```python
from build123d import *

# Parameters (mm, degrees)
SKETCH1_R                = 12.75
BOSS_EXTRUDE1_DEPTH      = 13
SKETCH2_R                = 3.3
BOSS_EXTRUDE2_DEPTH      = 1
SKETCH3_R                = 2.5
BOSS_EXTRUDE3_DEPTH      = 10.5
SKETCH4_R                = 5
BOSS_EXTRUDE4_DEPTH      = 2
BOSS_EXTRUDE5_START      = 10.5
SKETCH5_R                = 2.5
BOSS_EXTRUDE5_DEPTH      = 10.5
CHAMFER1_SIZE            = 1
BOSS_EXTRUDE6_REACH      = 32.42
BOSS_EXTRUDE6_END_RADIUS = 22.75
SKETCH6_R                = 2.2


with BuildPart() as part:
    # Sketch1 → Boss-Extrude1 (new body)
    with BuildSketch(Plane(origin=(0, 0, 0), x_dir=(1, 0, 0), z_dir=(0, 1, 0))):
        with Locations(Location((0, 0, 0), (0, 0, 90))):
            Circle(SKETCH1_R)
    extrude(amount=BOSS_EXTRUDE1_DEPTH)

    # Sketch2 → Boss-Extrude2 (add)
    with BuildSketch(Plane(origin=(0, 13, 0), x_dir=(1, 0, 0), z_dir=(0, 1, 0))):
        with Locations(Location((0, 0, 0), (0, 0, 270))):
            Circle(SKETCH2_R)
    extrude(amount=BOSS_EXTRUDE2_DEPTH)

    # Sketch3 → Boss-Extrude3 (add)
    with BuildSketch(Plane(origin=(0, 14, 0), x_dir=(1, 0, 0), z_dir=(0, 1, 0))):
        with Locations(Location((0, 0, 0), (0, 0, 90))):
            Circle(SKETCH3_R)
    extrude(amount=BOSS_EXTRUDE3_DEPTH)

    # Sketch4 → Boss-Extrude4 (add)
    with BuildSketch(Plane.XZ):
        with Locations(Location((0, 0, 0), (0, 0, 270))):
            Circle(SKETCH4_R)
    extrude(amount=BOSS_EXTRUDE4_DEPTH)

    # Sketch5 → Boss-Extrude5 (add)
    with BuildSketch(Plane.XZ.offset(2).offset(BOSS_EXTRUDE5_START)):
        with Locations(Location((0, 0, 0), (0, 0, 270))):
            Circle(SKETCH5_R)
    extrude(amount=-BOSS_EXTRUDE5_DEPTH)

    # Chamfer1
    chamfer1_edges = [part.edges().sort_by_distance(p)[0] for p in [
        (0, 24.5, 2.5),
        (0, -12.5, 2.5),
    ]]
    chamfer(chamfer1_edges, length=CHAMFER1_SIZE)

    # Boss-Extrude6: up to this cylinder (the profile starts inside it)
    boss_extrude6_end = Plane(origin=(0, 3.7, 0), z_dir=(0, -1, 0)) * Cylinder(BOSS_EXTRUDE6_END_RADIUS, 111.34, mode=Mode.PRIVATE)
    # Sketch6 → Boss-Extrude6 (add, up to the surface)
    with BuildSketch(Plane(origin=(0, 0, 0), x_dir=(0, 0, -1), z_dir=(1, 0, 0)), mode=Mode.PRIVATE) as boss_extrude6_sk1:
        with Locations(Location((0, 3.7, 0), (0, 0, 180))):
            Circle(SKETCH6_R)
    boss_extrude6_tool1 = extrude(boss_extrude6_sk1.sketch, amount=BOSS_EXTRUDE6_REACH, mode=Mode.PRIVATE) & boss_extrude6_end
    add(boss_extrude6_tool1.solids().sort_by_distance((0, 3.7, 0))[0])


solid = part.part
```
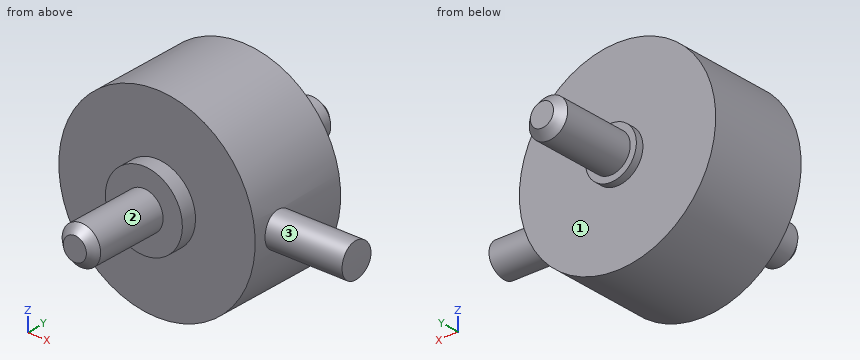
Model file for the job. Use its own axes, mm. Face numbers are marked on the shaded views. A direction names the side the tool comes from. Coordinates: 2 decimals unless noted, no trailing zeros. Order: outer loops, then holes, each group sorted by start corner. A loop starts at its lowest first (then second) coordinate and runs counter-clockwise, first axis right, second up. Notation, with made-up numbers: (-2.75, 71.25) -> (39.25, 71.25) arc R21 ccw to (39.25, 92.25) -> close; hole circle Ø9 at (41, -30). An arc over 180 degrees is marked (long way). Return JSON: item names as keys, results as strings.
Item 1: Slice it at B-B (x = 0). Write the cut outline in (y, z), then the cut area to 3 significant figures.
Model answer:
{"outline": "(-12.5, -1.5) -> (-11.5, -2.5) -> (-2, -2.5) -> (-2, -5) -> (0, -5) -> (0, -12.75) -> (13, -12.75) -> (13, -3.3) -> (14, -3.3) -> (14, -2.5) -> (23.5, -2.5) -> (24.5, -1.5) -> (24.5, 1.5) -> (23.5, 2.5) -> (14, 2.5) -> (14, 3.3) -> (13, 3.3) -> (13, 12.75) -> (0, 12.75) -> (0, 5) -> (-2, 5) -> (-2, 2.5) -> (-11.5, 2.5) -> (-12.5, 1.5) -> close", "area": "461 mm²"}
Item 2: Slice it at A-A (z = 0). Write the cut outline in (x, y), then the cut area to 3 significant figures.
Model answer:
{"outline": "(-12.75, 0) -> (-5, 0) -> (-5, -2) -> (-2.5, -2) -> (-2.5, -11.5) -> (-1.5, -12.5) -> (1.5, -12.5) -> (2.5, -11.5) -> (2.5, -2) -> (5, -2) -> (5, 0) -> (12.75, 0) -> (12.75, 1.5) -> (22.75, 1.5) -> (22.75, 5.9) -> (12.75, 5.9) -> (12.75, 13) -> (3.3, 13) -> (3.3, 14) -> (2.5, 14) -> (2.5, 23.5) -> (1.5, 24.5) -> (-1.5, 24.5) -> (-2.5, 23.5) -> (-2.5, 14) -> (-3.3, 14) -> (-3.3, 13) -> (-12.75, 13) -> close", "area": "505 mm²"}
Item 3: 3-axis set-ups, long thin cutter, end or side, ignore diameter. For the marked faces 1, 2 and 3: which of +Z, -Z, +X, -X, +Y, -Y reach the whole face in a straight line?
Model answer:
{"face 1": "+Y", "face 2": "-Y", "face 3": "+X"}
Item 4: Slice it at D-D (z = -4.5). Write the cut outline in (x, y), then the cut area to 3 significant figures.
Model answer:
{"outline": "(-11.93, 0) -> (-2.18, 0) -> (-2.18, -2) -> (2.18, -2) -> (2.18, 0) -> (11.93, 0) -> (11.93, 13) -> (-11.93, 13) -> close", "area": "319 mm²"}
Item 5: Pin check, flat tips, straight feed: P1, Ø3, axis at x = 0, z = -2, coming from the -Y side; P2, Ø6, axis at y = 16.5, z = 9.5, coming from the +X side; P3, Ø3, axis at y = 6.5, z = 2.5, coming from the +X side; P4, Ø4, axis at y = 4.5, z = -4.5, coming from the -X side. Stop position of each tip, or through.
Model answer:
{"P1": "stops at y = -12.5", "P2": "passes through", "P3": "stops at x = 12.71", "P4": "stops at x = -12.5"}
Item 6: Wall check: line 1 along Y through (x, z) = (-2.5, 7.5); line 2 along X through (y, z) = (-1, 3.5); line 3 along X through (y, z) = (12, -3.5). Give the ranges that are in metal, low to high. Write a range as from..to.
Model answer:
{"line 1": "y = 0..13", "line 2": "x = -3.57..3.57", "line 3": "x = -12.26..12.26"}
Item 7: Slice it at C-C (y = 3.7). Write the cut outline in (x, z), then the cut area to 3 significant figures.
Model answer:
{"outline": "(12.56, -2.2) -> (22.64, -2.2) arc R22.75 ccw to (22.64, 2.2) -> (12.56, 2.2) arc R12.75 ccw (long way) to start", "area": "555 mm²"}
